Here's how the part is built. I have some questions about the finished solid (model axes, mm). A direction names the side the tool comes from. Coordinates: 2 decimals unless noted, no trailing zeros. Loops run counter-clockwise (first coordinate to the right, second up) from the corner with the lowest first, then second, coordinate; pieces in that order, holes last. Notation, with made-up numbers: (-27.5, 81) -> (22.5, 81) arc R17 ccw to (22.5, 85) -> close; hole circle Ø4 at (75.5, -26.75). An arc over 180 degrees is marked (long way). Answer as a JSON object with one key per item and string values. Group by question number.
1) I want a section at C-C (z = 86.5). Write out the boundary of the cut face in (x, y).
2) I want a section at A-A (x = 0). Write out the boundary of the cut face in (y, z).
3) I want a section at D-D (x = -25). Write out the boundary of the cut face in (y, z), then the cut area to 3 significant figures.
4) I want a section at B-B (y = -69.5). Write out the boundary of the cut face in (x, z), then the cut area to 3 significant figures.
5) I'm going to push flat-ended pins straight in: pin 1 (7.5 mm diameter, centred on y = -71.5, z = 12, fed in from -X); pin 2 (9 mm diameter, centred on y = -33.5, z = 60, fed in from +X); pin 3 (1 mm diameter, centred on x = 15, y = -67.5, fed in from -Z); pin 4 (15 mm diameter, centred on y = -44, z = 69, fed in from -X). Where does each tip first touch, or does it pass through?
6) Which directions (+Z, -Z, +X, -X, +Y, -Y) give clear straight access to the entire face, cutting with the end or side of a thin tool? Please do faces 4 (the flat face through (50, -17, 54)), 5 (the flat face through (-10, -69, 13)), 6 (the flat face through (-20, -34, 44)).
7) If we mould it in two halves opening along X, with no side actions, what happens to faces 1 (the flat face through (8, -50, 25.4)), 2 (the cylindrical face through (-45.49, -51.16, 21.12)), 3 (the flat face through (25.07, -40.19, 58.355))? For each: +X half, -X half, draft (parallel to the pull), parting line (faces both ways), or undercut.
8) I need wall thicknesses on probe 1 along X at (y, z) = (-33, 45); probe 2 along Z at (x, y) = (0, -19); probe 3 along X at (y, z) = (-16, 137). Which ranges of each line are inside material? Lowest first, please. Write a range as [from, to].
```python
from build123d import *

# Parameters (mm, degrees)
F1_DEPTH = 50
F4_DEPTH = 25.401
F2_R     = 10
F5_DEPTH = 76.201
F8_DEPTH = 5
F11_R    = 15


# Not quite as in the source:
# - a feature of the source that left no trace in its solid (it failed there, or was rolled back) is left out
# - a pattern or mirror of a feature is missing from the dataset's text; its kind, count and spacing are read off the source's solid


with BuildPart() as f1:
    # F0 (on Right) → F1 (new body, symmetric)
    with BuildSketch(Plane.YZ):
        Polygon((-76.2, 0), (0, 0), (0, 152.4), (-25.4, 152.4), (-25.4, 25.4), (-76.2, 25.4), align=None)
    extrude(amount=F1_DEPTH, both=True)

    # F3 (on face) → F4 (cut, through all)
    with BuildSketch(Plane.XY.offset(25.4)):
        with BuildLine():
            ThreePointArc((-10, -61.2), (0, -71.2), (10, -61.2))
            ThreePointArc((10, -61.2), (0, -51.2), (-10, -61.2))
        make_face()
        with BuildLine():
            Line((10, -76.2), (10, -61.2))
            ThreePointArc((10, -61.2), (0, -71.2), (-10, -61.2))
            Line((-10, -61.2), (-10, -76.2))
            Line((-10, -76.2), (10, -76.2))
        make_face()
    extrude(amount=-F4_DEPTH, mode=Mode.SUBTRACT)

    # F2 (on face) → F5 (cut, through all)
    with BuildSketch(Plane(origin=(0, 0, 0), x_dir=(-1, 0, 0), z_dir=(0, 1, 0))):
        with Locations((0, 137.4)):
            Circle(F2_R)
    extrude(amount=-F5_DEPTH, mode=Mode.SUBTRACT)

    # F7 (on offset) → F8 (join, symmetric)
    with BuildSketch(Plane.YZ.offset(25)):
        Polygon((-25.4, 25.4), (-25.4, 90.4), (-55.4, 25.4), align=None)
    f8 = extrude(amount=F8_DEPTH, both=True)

    # F8_copies: F8 across plane
    add(f8.mirror(Plane(origin=(0, 0, 0), x_dir=(0, 0, -1), z_dir=(-1, 0, 0))))

    # F11 (call 1 of 5: OpenCascade refuses the feature's edges together)
    f11_edges = [f1.edges().sort_by_distance(p)[0] for p in [
        (-50, -12.7, 152.4),
    ]]
    fillet(f11_edges, radius=F11_R)

    # F11#2 (call 2 of 5)
    f11_2_edges = [f1.edges().sort_by_distance(p)[0] for p in [
        (50, -12.7, 152.4),
    ]]
    fillet(f11_2_edges, radius=F11_R)

    # F11#3 (call 3 of 5)
    f11_3_edges = [f1.edges().sort_by_distance(p)[0] for p in [
        (0, 0, 0),
    ]]
    fillet(f11_3_edges, radius=F11_R)

    # F11#4 (call 4 of 5)
    f11_4_edges = [f1.edges().sort_by_distance(p)[0] for p in [
        (50, -76.2, 12.7),
    ]]
    fillet(f11_4_edges, radius=F11_R)

    # F11#5 (call 5 of 5)
    f11_5_edges = [f1.edges().sort_by_distance(p)[0] for p in [
        (-50, -76.2, 12.7),
        (-50, -50.8, 25.4),
    ]]
    fillet(f11_5_edges, radius=F11_R)


solid = f1.part
```
Determined:
{
 "1": {"outline": "(-50, -25.4) -> (-30, -25.4) -> (-30, -27.2) -> (-20, -27.2) -> (-20, -25.4) -> (20, -25.4) -> (20, -27.2) -> (30, -27.2) -> (30, -25.4) -> (50, -25.4) -> (50, 0) -> (-50, 0) -> close"},
 "2": {"outline": "(-51.2, 0) -> (-15, 0) arc R15 ccw to (0, 15) -> (0, 127.4) -> (-25.4, 127.4) -> (-25.4, 25.4) -> (-51.2, 25.4) -> close; (-25.4, 147.4) -> (0, 147.4) -> (0, 152.4) -> (-25.4, 152.4) -> close"},
 "3": {"outline": "(-76.2, 0) -> (-15, 0) arc R15 ccw to (0, 15) -> (0, 152.4) -> (-25.4, 152.4) -> (-25.4, 90.4) -> (-55.4, 25.4) -> (-76.2, 25.4) -> close", "area": "6,090 mm^2"},
 "4": {"outline": "(-47.49, 0) -> (-10, 0) -> (-10, 25.4) -> (-35, 25.4) arc R15 ccw to (-47.49, 18.7) -> close; (10, 0) -> (47.49, 0) -> (47.49, 25.4) -> (10, 25.4) -> close", "area": "1,880 mm^2"},
 "5": {"pin 1": "x = -48.49", "pin 2": "x = 30", "pin 3": "z = 0", "pin 4": "through"},
 "6": {"face 4": "+Z, -Z, +X, +Y, -Y", "face 5": "+Z, -Z, -Y", "face 6": "+Z, -Y"},
 "7": {"face 1": "undercut", "face 2": "-X half", "face 3": "draft"},
 "8": {"probe 1": "[-30, -20], [20, 30]", "probe 2": "[0, 127.4], [147.4, 152.4]", "probe 3": "[-50, -9.99], [9.99, 50]"}
}
